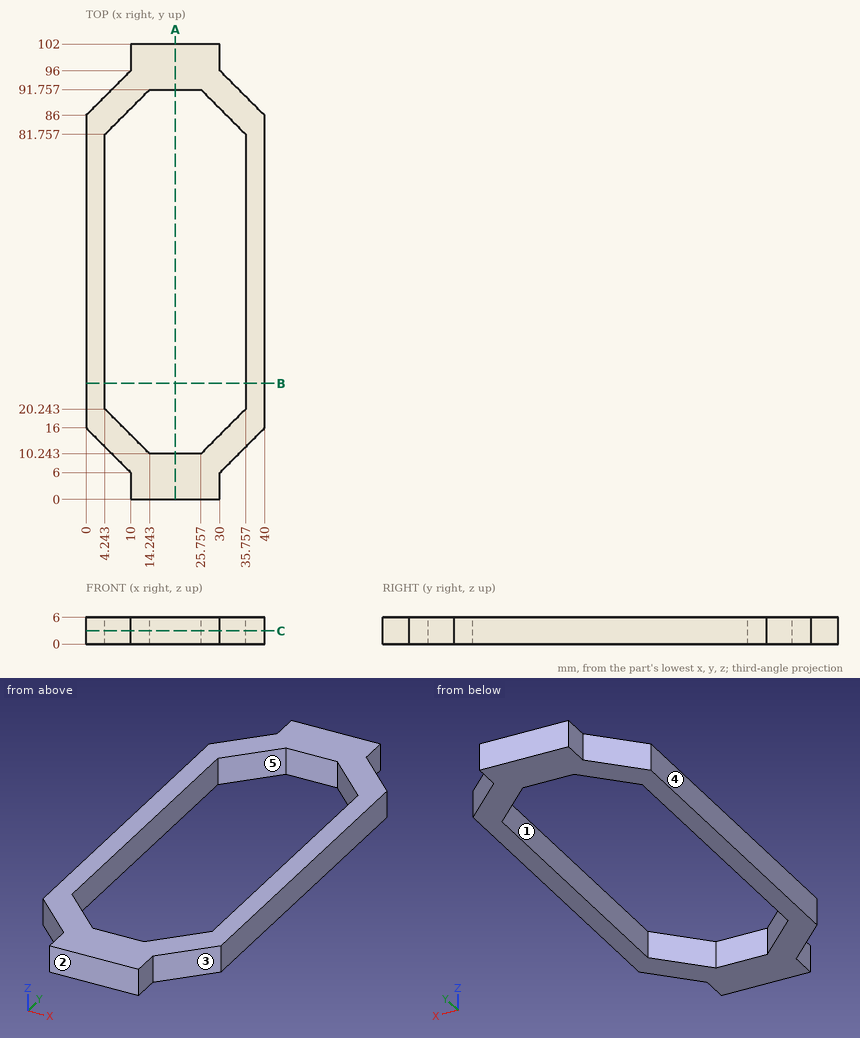
Answer from the drawing. Dimensions are ordinates in mm from the lowest x, y and z of the part. A direction names the side the tool comes from. Give positions to 0.01 mm unless a question says otherwise; leave off trailing zeros. Write each loop counter-clockwise with the first axis right and the second up, starting at its lowest first coordinate (ties: lowest second). Pieces come first, ordered by that corner, then holes. Notation, with made-up numbers: (71.25, 51) - (129.25, 51) arc R24 ccw to (129.25, 73) - close; hole circle Ø8 at (1.5, 75). An arc over 180 degrees is marked (long way). One line per item, written item: value. Start each with the question number.
1. Consider probe 1 along X at (y, z) = (75, 4.75); probe 2 along Y at (x, z) = (23, 3.1); probe 3 along Y at (x, z) = (8, 1.5) (1 decimal). Determine where each line is inside the solid, lowest interval first.
2. Find section C-C (z = 3). Write down the section's boundary in (x, y), then the cut area to 3 significant figures.
3. Find section B-B (y = 26). Write down the section's boundary in (x, z), then the cut area to 3 significant figures.
4. For a pull along X with two mould halves and no side action, classify the marked faces 3, 4 and 5 as +X half, -X half, draft (parallel to the pull), parting line (faces both ways), or undercut.
5. For the marked faces 1 and 2, determine the directions among +Z, -Z, +X, -X, +Y, -Y from which every point of the face is accessible in a straight line to the end or side of a thin tool.
6. Given pin 1 (1.8 mm diameter, centred on y = 4, z = 4.5, fed in from +X); pin 2 (1.8 mm diameter, centred on y = 3, z = 2.5, fed in from -X), each flat-ended and moving along its own axis, determine where each tip first touches the part or whether it passes through.
7. Find section A-A (x = 20). Write down the section's boundary in (y, z), then the cut area to 3 significant figures.
Geometry results:
1. probe 1: 0 to 4.24, 35.76 to 40
1. probe 2: 0 to 10.24, 91.76 to 102
1. probe 3: 8 to 16.5, 85.5 to 94
2. outline: (0, 16) - (10, 6) - (10, 0) - (30, 0) - (30, 6) - (40, 16) - (40, 86) - (30, 96) - (30, 102) - (10, 102) - (10, 96) - (0, 86) - close; hole (4.24, 20.24) - (14.24, 10.24) - (25.76, 10.24) - (35.76, 20.24) - (35.76, 81.76) - (25.76, 91.76) - (14.24, 91.76) - (4.24, 81.76) - close
2. area: 1,270 mm2
3. outline: (0, 0) - (4.24, 0) - (4.24, 6) - (0, 6) - close; (35.76, 0) - (40, 0) - (40, 6) - (35.76, 6) - close
3. area: 50.9 mm2
4. face 3: +X half
4. face 4: -X half
4. face 5: undercut
5. face 1: +Z, -Z
5. face 2: +Z, -Z, +X, -X, -Y
6. pin 1: x = 30
6. pin 2: x = 10
7. outline: (0, 0) - (10.24, 0) - (10.24, 6) - (0, 6) - close; (91.76, 0) - (102, 0) - (102, 6) - (91.76, 6) - close
7. area: 123 mm2
